from build123d import *

# Parameters (mm, degrees)
SKETCH1_W           = 90
SKETCH1_H           = 20
BOSS_EXTRUDE2_DEPTH = 16
SKETCH2_R           = 1.5
CUT_EXTRUDE1_DEPTH  = 16
SKETCH3_W           = 110.03675272
SKETCH3_H           = 13
CUT_EXTRUDE2_DEPTH  = 23
SKETCH4_R           = 3
BOSS_EXTRUDE3_DEPTH = 16


with BuildPart() as part:
    # Sketch1 → Boss-Extrude2 (new body)
    with BuildSketch(Plane.XY):
        with BuildLine():
            Line((-3.745126611, 2.099543411), (-3.745126611, -17.900456589))
            ThreePointArc((-3.745126611, -17.900456589), (-13.745126611, -7.900456589), (-3.745126611, 2.099543411))
        make_face()
        with Locations((41.254873389, -7.900456589)):
            Rectangle(SKETCH1_W, SKETCH1_H)
        with BuildLine():
            ThreePointArc((86.254873389, 2.099543411), (96.254873389, -7.900456589), (86.254873389, -17.900456589))
            Line((86.254873389, -17.900456589), (86.254873389, 2.099543411))
        make_face()
    extrude(amount=BOSS_EXTRUDE2_DEPTH)

    # Sketch2 → Cut-Extrude1 (cut)
    with BuildSketch(Plane.XY.offset(16)):
        with Locations((-3.745126611, -7.900456589)):
            Circle(SKETCH2_R)
        with Locations((86.254873389, -7.900456589)):
            Circle(SKETCH2_R)
    extrude(amount=-CUT_EXTRUDE1_DEPTH, mode=Mode.SUBTRACT)

    # Sketch3 → Cut-Extrude2 (cut)
    with BuildSketch(Plane(origin=(0, 2.099543411, 0), x_dir=(1, 0, 0), z_dir=(0, 1, 0))):
        with Locations((41.257830101, -8)):
            Rectangle(SKETCH3_W, SKETCH3_H)
    extrude(amount=-CUT_EXTRUDE2_DEPTH, mode=Mode.SUBTRACT)

    # Sketch4 → Boss-Extrude3 (add)
    with BuildSketch(Plane(origin=(0, 0, 0), x_dir=(-1, 0, 0), z_dir=(0, 0, -1))):
        with Locations((-36.254873389, -7.900456589)):
            Circle(SKETCH4_R)
        with Locations((-46.254873389, -7.900456589)):
            Circle(SKETCH4_R)
    extrude(amount=-BOSS_EXTRUDE3_DEPTH)


solid = part.part
The model under review builds one solid part; all positions refer to its coordinate system, in mm. A direction names the side the tool comes from. Round coordinates to 2 decimals unless told otherwise and drop trailing zeros. Order: outer loops, then holes, each group sorted by start corner. A loop starts at its lowest first (then second) coordinate and runs counter-clockwise, first axis right, second up. Notation, with made-up numbers: (-10.5, 17.5) -> (31.5, 17.5) arc R5 cw to (31.5, 22.5) -> close; hole circle Ø7 at (88, 7.5). An arc over 180 degrees is marked (long way). Write item = value, one per line. Start each with the question number.
Item 1: Mouldability with a two-part tool opening along Y and no side actions: class faces 1 (the face through (84.756, -7.835, 15.26)), 2 (the face through (-13.743, -8.12, 15.24)), 3 (the face through (42, -8, 0)) as released by +Y, released by -Y, zero draft, split by the parting line, or undercut.
Item 2: For line 1 along Z through (x, y) = (16.5, -2.75); line 2 along X through (y, z) = (-7.75, 7); line 3 along X through (y, z) = (-6.75, 2.75), list the stretches that pass through material, from the lowest coordinate up.
Item 3: Consider section A-A on y = -2.75. Write out the cut boundary in (x, z), plus the area to 3 significant figures.
Item 4: Consider section B-B on x = 11. Write out the cut boundary in (y, z).
Item 5: Clearance check with flat-ended pins moving along their axes: pin 1 Ø2 at (x, z) = (48.5, 9.5) entering from -Y; pin 2 Ø2 at (y, z) = (-11, 9.5) entering from -X; pin 3 Ø1 at (x, z) = (46.5, 13) entering from -Y; pin 4 Ø2.5 at (x, y) = (86.25, -7.9) entering from -Z. State where each tip first meets the part, or that it passes through.
Item 6: Consider section C-C on z = 10.75. Write out the cut boundary in (x, y).
Item 7: For faces 4 (the face through (43.393, -6.999, 7.909)), 5 (the face through (84.756, -7.835, 0.761)), list the 3-axis set-ups (+Z, -Z, +X, -X, +Y, -Y) from which the entire face can be reached by the end or side of a thin tool; tool diameter is ignored.
Conclusion:
q1.face_1 = undercut
q1.face_2 = split by the parting line
q1.face_3 = zero draft
q2.line_1 = 0 to 1.5, 14.5 to 16
q2.line_2 = 33.26 to 39.25, 43.26 to 49.25
q2.line_3 = 33.48 to 39.03, 43.48 to 49.03
q3.outline = (-12.32, 0) -> (94.83, 0) -> (94.83, 1.5) -> (-12.32, 1.5) -> close; (-12.32, 14.5) -> (94.83, 14.5) -> (94.83, 16) -> (-12.32, 16) -> close
q3.area = 321 mm2
q4.outline = (-17.9, 0) -> (2.1, 0) -> (2.1, 1.5) -> (-17.9, 1.5) -> close; (-17.9, 14.5) -> (2.1, 14.5) -> (2.1, 16) -> (-17.9, 16) -> close
q5.pin_1 = -10.63
q5.pin_2 = 34.11
q5.pin_3 = -10.9
q5.pin_4 = through
q6.outline = circle Ø6 at (36.25, -7.9); circle Ø6 at (46.25, -7.9)
q7.face_4 = none
q7.face_5 = +Z, -Z
